Design review of the part built by this model. Coordinates are the model's own, in mm. Give positions to 0.01 mm unless a question says otherwise; leave off trailing zeros. Write each loop counter-clockwise with the first axis right and the second up, starting at its lowest first coordinate (ties: lowest second). Pieces come first, ordered by that corner, then holes. Notation, with made-up numbers: (-36.75, 55.25) - (-3.75, 55.25) arc R13 ccw to (-3.75, 63.25) - close; hole circle Ø3 at (43, -0.5). An arc over 180 degrees is marked (long way). Use a Markdown table: item, result. Add a question column.
```python
from build123d import *

# Parameters (mm, degrees)
F1_DEPTH = 825.5


with BuildPart() as f1:
    # F0 (on Right) → F1 (new body, symmetric)
    with BuildSketch(Plane.YZ):
        with BuildLine():
            Line((-17.4017421393, 5.936837718), (-52.8176613152, 2.3044354748))
            Line((-52.8176613152, 2.3044354748), (-52.8176613152, 0))
            Line((-52.8176613152, 0), (55.627758292, 0))
            Line((55.627758292, 0), (55.627758292, 31.5129175921))
            Line((55.627758292, 31.5129175921), (50.5852726164, 28.3613643292))
            ThreePointArc((50.5852726164, 28.3613643292), (34.4368278859, 19.8181329), (17.22969466, 13.6802475466))
            Line((17.22969466, 13.6802475466), (3.594874024, 9.8971762013))
            ThreePointArc((3.594874024, 9.8971762013), (-6.8199988392, 7.474656574), (-17.4017421393, 5.936837718))
        make_face()
    extrude(amount=F1_DEPTH, both=True)


solid = f1.part
```
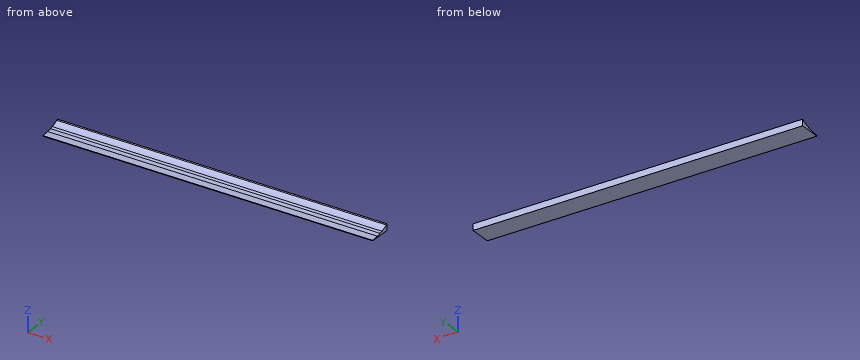
(1) Insertion check: pin 1 (6 mm diameter, centred on x = -572.5, y = -37, fed in from -Z). The pin has a flat end and moves straight along its axis. Give the tip position at first contact, or say it passes through.
(2) Add section B-B (z = 18.5). State the section outline as (x, y) points.
(3) Add section A-A (x = 354.5). State the section outline as (y, z) points.
(4) Add section C-C (y = -38.5). State the section outline as (x, z) points.
(5) For line 1 along Z through (x, y) = (333.5, -40.5); line 2 along Z through (x, y) = (-291.5, 33.5); line 3 along Y through (x, z) = (-589, 24.5), list the stretches that pass through material, from the lowest coordinate up.
Answers follow:
| question | item | result |
|---|---|---|
| 1 | pin 1 | z = 0 |
| 2 | outline | (-825.5, 31.33) - (825.5, 31.33) - (825.5, 55.63) - (-825.5, 55.63) - close |
| 3 | outline | (-52.82, 0) - (55.63, 0) - (55.63, 31.51) - (50.59, 28.36) arc R127 cw to (17.23, 13.68) - (3.59, 9.9) arc R127 cw to (-17.4, 5.94) - (-52.82, 2.3) - close |
| 4 | outline | (-825.5, 0) - (825.5, 0) - (825.5, 3.77) - (-825.5, 3.77) - close |
| 5 | line 1 | 0 to 3.57 |
| 5 | line 2 | 0 to 19.41 |
| 5 | line 3 | 43.97 to 55.63 |
